The model under review builds one solid part; all positions refer to its coordinate system, in mm. Face numbers are marked on the shaded views. A direction names the side the tool comes from. Coordinates: 2 decimals unless noted, no trailing zeros. Write each loop counter-clockwise with the first axis right and the second up, starting at its lowest first coordinate (ties: lowest second). Pieces come first, ordered by that corner, then holes.
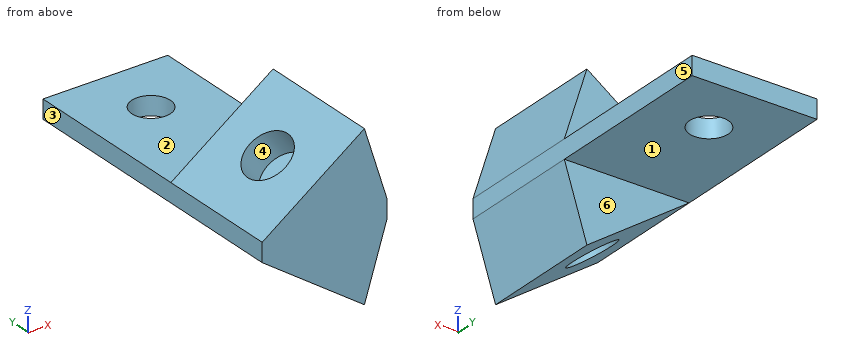
```python
from build123d import *

# Parameters (mm, degrees)
F0_W     = 20
F0_H     = 48
F1_DEPTH = 3
F2_R     = 3.1
F3_DEPTH = 25
F5_DEPTH = 20
F6_R     = 3.9
F7_DEPTH = 5
F8_R     = 3.9
F9_DEPTH = 5


with BuildPart() as f1:
    # F0 (on Top) → F1 (new body)
    with BuildSketch(Plane.XY):
        Rectangle(F0_W, F0_H)
    extrude(amount=F1_DEPTH)

    # F2 (on face) → F3 (cut)
    with BuildSketch(Plane.XY.offset(3)):
        with Locations((0, 14)):
            Circle(F2_R)
    extrude(amount=-F3_DEPTH, mode=Mode.SUBTRACT)

    # F4 (on face) → F5 (join)
    with BuildSketch(Plane.XZ.offset(24)):
        Polygon((6.3830408858, 14.471528727), (-10, 3), (10, 3), align=None)
        Polygon((10, 0), (-10, 0), (6.3830408858, -11.471528727), align=None)
    extrude(amount=-F5_DEPTH)

    # F6 (on face) → F7 (cut)
    with BuildSketch(Plane(origin=(-4.6994382146, 0, 6.7114933189), x_dir=(0.8191520443, 0, 0.5735764364), z_dir=(-0.5735764364, 0, 0.8191520443))):
        with Locations((3.5292088662, -14)):
            Circle(F6_R)
    extrude(amount=-F7_DEPTH, mode=Mode.SUBTRACT)

    # F8 (on face) → F9 (cut)
    with BuildSketch(Plane(origin=(-3.2898992834, 0, -4.6984631039), x_dir=(0.8191520443, 0, -0.5735764364), z_dir=(-0.5735764364, 0, -0.8191520443))):
        with Locations((1.8084795571, 14)):
            Circle(F8_R)
    extrude(amount=-F9_DEPTH, mode=Mode.SUBTRACT)


solid = f1.part
```
Item 1: For pin 1 (5.5 mm diameter, centred on x = 4.5, z = 9, fed in from +Y); pin 2 (2 mm diameter, centred on x = 0, y = 9.5, fed in from -Z); pin 3 (5 mm diameter, centred on y = -18, z = -7.5, fed in from -X), all flat-tipped, find the tip position at first contact; note any pin that passes through.
Solved:
pin 1: stops at y = -4
pin 2: stops at z = 0
pin 3: stops at x = -2.86
Item 2: Take a section at A-A, the plane y = 14. Write out the cut boundary in (x, z).
Solved:
outline: (-10, 0) - (-3.1, 0) - (-3.1, 3) - (-10, 3) - close; (3.1, 0) - (10, 0) - (10, 3) - (3.1, 3) - close
Item 3: To check wall thickness, follow line 1 along Y through (x, z) = (0, 0.8); line 2 along Y through (x, z) = (7.75, 6.75); line 3 along Y through (x, z) = (0.5, -5.25). State the ranges of each line that lie inside material, in increasing order.
Solved:
line 1: y = -24 to 10.9, 17.1 to 24
line 2: y = -24 to -4
line 3: y = -24 to -17.55, -10.45 to -4
Item 4: Mouldability with a two-part tool opening along Y and no side actions: class the marked faces 4, 5 and 6 as pulls with the +Y half, pulls with the -Y half, needs draft (parallel to the pull), parting line crosses it, or undercut.
Solved:
face 4: undercut
face 5: needs draft
face 6: pulls with the +Y half
Item 5: Machinability: for the marked faces 1, 2 and 3, which of the approach directions +Z, -Z, +X, -X, +Y, -Y give a long, thin tool a straight path to every point of the face, cutting with its end or side? Answer none if there is none.
Solved:
face 1: -Z, +X, -X, +Y
face 2: +Z, +X, -X, +Y
face 3: +Z, -Z, -X, +Y, -Y
Item 6: Take a section at C-C, the plane y = -9.5. Write out the cut boundary in (x, z).
Solved:
outline: (-10, 0) - (6.38, -11.47) - (10, 0) - (10, 3) - (6.38, 14.47) - (-10, 3) - close
Item 7: Take a section at D-D, the plane x = 8.25. Write out the cut boundary in (y, z).
Solved:
outline: (-24, -5.55) - (-4, -5.55) - (-4, 0) - (24, 0) - (24, 3) - (-4, 3) - (-4, 8.55) - (-24, 8.55) - close
Item 8: Take a section at B-B, the plane z = 1.25. Write out the cut boundary in (x, y).
Solved:
outline: (-10, -24) - (10, -24) - (10, 24) - (-10, 24) - close; hole circle Ø6.2 at (0, 14)
